from build123d import *

# Parameters (mm, degrees)
EXTRUDE_1_DEPTH     = 27
SKETCH_3_R          = 2
EXTRUDE_2_DEPTH     = 2.5
EXTRUDE_3_DEPTH     = 8.5
SKETCH_5_W          = 33.531111889
SKETCH_5_H          = 20
EXTRUDE_4_DEPTH     = 2
FILLET_5_R          = 2
SKETCH_6_R          = 5
EXTRUDE_5_DEPTH     = 2
FILLET_7_R          = 1
SKETCH_7_R          = 2.9
CUT_EXTRUDE_1_DEPTH = 27
RIB_8_REACH         = 41.472
SKETCH_8_WALL_W     = 88.288518024
SKETCH_8_WALL_H     = 2


with BuildPart() as part:
    # 草图2 → 凸台-拉伸1 (new body)
    with BuildSketch(Plane(origin=(0, 0, 0), x_dir=(1, 0, 0), z_dir=(0, 1, 0))):
        Polygon((0, -10), (-20, -10), (-20, 10), (20, 10), (20, -10), align=None)
    extrude(amount=-EXTRUDE_1_DEPTH)

    # 草图3 → 凸台-拉伸2 (add)
    with BuildSketch(Plane(origin=(0, 0, 0), x_dir=(1, 0, 0), z_dir=(0, 1, 0))):
        Polygon((0, 10), (27, 10), (27, -10), (-27, -10), (-27, 10), align=None)
        with Locations(Location((-24.315, -5, 0), (0, 0, 270))):
            Circle(SKETCH_3_R, mode=Mode.SUBTRACT)
        with Locations(Location((-24.315, 5, 0), (0, 0, 90))):
            Circle(SKETCH_3_R, mode=Mode.SUBTRACT)
        with Locations(Location((24.315, -5, 0), (0, 0, 90))):
            Circle(SKETCH_3_R, mode=Mode.SUBTRACT)
        with Locations(Location((24.315, 5, 0), (0, 0, 270))):
            Circle(SKETCH_3_R, mode=Mode.SUBTRACT)
    extrude(amount=EXTRUDE_2_DEPTH)

    # 草图4 → 凸台-拉伸3 (add)
    with BuildSketch(Plane(origin=(0, 2.5, 0), x_dir=(1, 0, 0), z_dir=(0, 1, 0))):
        Polygon((0, 10), (-20, 10), (-20, -10), (20, -10), (20, 10), align=None)
    extrude(amount=EXTRUDE_3_DEPTH)

    # 草图5 → 凸台-拉伸4 (add)
    with BuildSketch(Plane(origin=(0, 11, 0), x_dir=(1, 0, 0), z_dir=(0, 1, 0))):
        with Locations((-3.234444055, 0)):
            Rectangle(SKETCH_5_W, SKETCH_5_H)
    extrude(amount=EXTRUDE_4_DEPTH)

    # 圆角5
    fillet_5_edges = [part.edges().sort_by_distance(p)[0] for p in [
        (13.531111889, 13, 0),
    ]]
    fillet(fillet_5_edges, radius=FILLET_5_R - 0.0001)  # a hair under: the kernel refuses the full size

    # 草图6 → 凸台-拉伸5 (add)
    with BuildSketch(Plane(origin=(0, 13, 0), x_dir=(1, 0, 0), z_dir=(0, 1, 0))):
        with Locations(Location((-9.85, 0, 0), (0, 0, 90))):
            Circle(SKETCH_6_R)
    extrude(amount=EXTRUDE_5_DEPTH)

    # 圆角7
    fillet_7_edges = [part.edges().sort_by_distance(p)[0] for p in [
        (-9.85, 15, 5),
    ]]
    fillet(fillet_7_edges, radius=FILLET_7_R)

    # 草图7 → 切除-拉伸1 (cut)
    with BuildSketch(Plane(origin=(0, 15, 0), x_dir=(1, 0, 0), z_dir=(0, 1, 0))):
        with Locations(Location((-9.85, 0, 0), (0, 0, 270))):
            Circle(SKETCH_7_R)
    extrude(amount=-CUT_EXTRUDE_1_DEPTH, mode=Mode.SUBTRACT)

    # 草图8 wall → 筋8 (add, up to next)
    with BuildSketch(Plane(origin=(-23.5, 3.613146338, 0), x_dir=(0.952964322003, 0.303082498652, 0), z_dir=(-0.303082498652, 0.952964322003, 0)), mode=Mode.PRIVATE) as rib_8_sk1:
        Rectangle(SKETCH_8_WALL_W, SKETCH_8_WALL_H)
    rib_8_tool1 = extrude(rib_8_sk1.sketch, amount=-RIB_8_REACH, mode=Mode.PRIVATE) - part.part
    rib_8 = rib_8_tool1.solids().sort_by_distance((-23.5, 3.613146338, 0))[0]
    add(rib_8)

    # 镜向1: 筋8 across plane
    add(rib_8.mirror(Plane(origin=(0, 0, 0), x_dir=(0, 0, 1), z_dir=(1, 0, 0))))


solid = part.part
Source: CAD feature listing. Evaluate the final solid. Frame: model axes, mm. A direction names the side the tool comes from. Round coordinates to 2 decimals unless told otherwise and drop trailing zeros. Order: outer loops, then holes, each group sorted by start corner. A loop starts at its lowest first (then second) coordinate and runs counter-clockwise, first axis right, second up. Notation, with made-up numbers: (11, -28.75) - (38, -28.75) arc R29 ccw to (38, 1.25) - close; hole circle Ø11 at (85, -7). An arc over 180 degrees is marked (long way). Use a Markdown table: item, result. Add a question column.
1. Line query: probe 1 along X at (y, z) = (0.6, -5) (3 decimals); probe 2 along X at (y, z) = (-14.5, -7.5); probe 3 along Y at (x, z) = (-0.5, 8). Output: solid intervals per line, ascending.
2. Set-up query: faces 1 (the cylindrical face through (-7.89, 1.69, -2.14)), 2 (the flat face through (22, 2.5, 5)), 3 (the flat face through (-27, 1, 0)), 4 (the flat face through (-22.67, 2.5, 6.44)), 5 (the flat face through (23.549, 3.598, -0.014)). Return all of +Z, -Z, +X, -X, +Y, -Y with unobstructed straight access to the full face (end or side cutting, diameter ignored); none if empty.
3. Section query B-B (y = -8). Return the cut outline in (x, z), then the cut area to 3 significant figures.
4. First-contact query: pin 1 (4.5 mm diameter, centred on x = -9.85, z = 0, fed in from +Y); pin 2 (2 mm diameter, centred on x = 24.5, z = -1.5, fed in from -Y); pin 3 (5 mm diameter, centred on y = -21, z = 3, fed in from -X); pin 4 (3 mm diameter, centred on x = 24.315, z = 5, fed in from +Y). Flat tips, straight axial feed; report the tip coordinate or a pass-through.
5. Mould query, pull axis Z, two halves, no side actions, for faces 6 (the cylindrical face through (-14.066, 13.493, -2.688)), 7 (the flat face through (0, -27, 0)), 8 (the cylindrical face through (-24.4, 1.2, -3)). Classes: +Z half, -Z half, draft (parallel to the pull), parting line (faces both ways), or undercut.
6. Section query C-C (x = -9.85). Return the cut outline in (y, z), then the cut area to 3 significant figures.
7. Section query D-D (y = 1). Return the cut outline in (x, z) (3 decimals).
Derived:
| question | item | result |
|---|---|---|
| 1 | probe 1 | -27 to -26.315, -22.315 to 22.315, 26.315 to 27 |
| 1 | probe 2 | -20 to 20 |
| 1 | probe 3 | -27 to 13 |
| 2 | face 1 | +Y |
| 2 | face 2 | +Z, +X, +Y |
| 2 | face 3 | +Z, -Z, -X, +Y, -Y |
| 2 | face 4 | +Z, -X, +Y |
| 2 | face 5 | +Z, -Z, +X, +Y |
| 3 | outline | (-20, -10) - (20, -10) - (20, 10) - (-20, 10) - close; hole circle Ø5.8 at (-9.85, 0) |
| 3 | area | 774 mm2 |
| 4 | pin 1 | y = -12 |
| 4 | pin 2 | y = 0 |
| 4 | pin 3 | x = -20 |
| 4 | pin 4 | through |
| 5 | face 6 | parting line |
| 5 | face 7 | draft |
| 5 | face 8 | undercut |
| 6 | outline | (-27, -10) - (13, -10) - (13, -5) - (14, -5) arc R1 ccw to (15, -4) - (15, -2.9) - (-12, -2.9) - (-12, 2.9) - (15, 2.9) - (15, 4) arc R1 ccw to (14, 5) - (13, 5) - (13, 10) - (-27, 10) - close |
| 6 | area | 663 mm2 |
| 7 | outline | (-27, -10) - (27, -10) - (27, 10) - (-27, 10) - close; hole circle Ø4 at (-24.315, -5); hole circle Ø4 at (-24.315, 5); hole circle Ø5.8 at (-9.85, 0); hole circle Ø4 at (24.315, -5); hole circle Ø4 at (24.315, 5) |
